Input: part model. Units: mm. Frame: model coordinates. A direction names the side the tool comes from. Round coordinates to 2 decimals unless told otherwise and drop trailing zeros. Write each loop counter-clockwise with the first axis right and the second up, starting at its lowest first coordinate (ties: lowest second). Pieces come first, ordered by that corner, then holes. Notation, with made-up numbers: (68, 26.5) -> (77, 26.5) arc R33 ccw to (77, 58.5) -> close; hole circle Ø10 at (68, 43.5). An arc over 180 degrees is marked (long way). Write item = value, one per line. Start each with the question number.
```python
from build123d import *

# Parameters (mm, degrees)
SHAFTSKETCH_R           = 6.5
BEARINGHOLEPAD_DEPTH    = 5
SHAFT1SKETCH_R          = 7.5
OBJ1 = 5
PIN1SKETCH_R            = 2
PIN1PAD_DEPTH           = 10
PIN2SKETCH_R            = 2
PIN2PAD_DEPTH           = 10
OBJ2    = 15


with BuildPart() as part:
    # ShaftSketch → bearingholePad (new body)
    with BuildSketch(Plane.XY):
        Circle(SHAFTSKETCH_R)
    extrude(amount=BEARINGHOLEPAD_DEPTH)

    with BuildSketch(Plane.XY.offset(5)):
        Circle(SHAFT1SKETCH_R)
    extrude(amount=OBJ1)

    # Pin1Sketch → Pin1Pad (join)
    with BuildSketch(Plane.XY.offset(5)):
        with Locations((1.75, 0)):
            Circle(PIN1SKETCH_R)
    extrude(amount=PIN1PAD_DEPTH)

    # Pin2Sketch → Pin2Pad (join)
    with BuildSketch(Plane.XY.offset(5)):
        with Locations((3.5, 0)):
            Circle(PIN2SKETCH_R)
    extrude(amount=PIN2PAD_DEPTH)

    with BuildSketch(Plane.XY):
        with BuildLine():
            ThreePointArc((-0.979796, 2.3), (0, -2.5), (0.979796, 2.3))
            Line((-0.979796, 2.3), (0.979796, 2.3))
        make_face()
    extrude(amount=OBJ2, mode=Mode.SUBTRACT)


solid = part.part
```
1. Section A-A (y = 0). Output: boundary loops of the cut face in (x, z).
2. Pin query (flat end, axial travel): P1, Ø6.5, axis at x = 0, y = 0, coming from the +Z side; P2, Ø3, axis at x = 5.5, z = 12, coming from the -Y side; P3, Ø1.6, axis at x = 0, z = 4, coming from the -Y side; P4, Ø5, axis at x = -0.5, z = 13, coming from the +Y side. Return the tip coordinate at first contact, or that it passes through.
3. Line query: line 1 along Y through (x, z) = (0, 9.75); line 2 along Y through (x, z) = (0, 4.5); line 3 along Z through (x, y) = (-4.75, 3). Output: solid intervals per line, ascending.
4. Section D-D (x = -6). Output: boundary loops of the cut face in (y, z), then the cut area to 3 significant figures.
5. Reachability of faces 4 (the cylindrical face through (2.077, -1.973, 12.465)), 5 (the cylindrical face through (-5.158, -3.955, 2.465)), 6 (the cylindrical face through (2.09, 1.97, 12.46)), 7 (the flat face through (0, 2.3, 5)) from +Z, -Z, +X, -X, +Y, -Y: full face, straight path, thin tool, end or side. Return the list, or none.
6. Section C-C (z = 7.5). Output: boundary loops of the cut face in (x, y).
7. Section B-B (x = 0). Output: boundary loops of the cut face in (y, z).
8. Mould query, pull axis Y, two halves, no side actions, for faces 1 (the cylindrical face through (5.5, -0.06, 12.46)), 2 (the cylindrical face through (2.31, -0.955, 5.728)), 3 (the flat face through (3, 0, 0)). Classes: pulls with the +Y half, pulls with the -Y half, needs draft (parallel to the pull), parting line crosses it, or undercut.
Check sheet entries:
q1.outline = (-7.5, 5) -> (-6.5, 5) -> (-6.5, 0) -> (-2.5, 0) -> (-2.5, 10) -> (-7.5, 10) -> close; (2.5, 0) -> (6.5, 0) -> (6.5, 5) -> (7.5, 5) -> (7.5, 10) -> (5.5, 10) -> (5.5, 15) -> (2.5, 15) -> close
q2.P1 = 15
q2.P2 = -1.94
q2.P3 = -6.5
q2.P4 = 2
q3.line_1 = -7.5 to -2.5, 2.3 to 7.5
q3.line_2 = -6.5 to -2.5, 2.3 to 6.5
q3.line_3 = 0 to 10
q4.outline = (-4.5, 5) -> (-2.5, 5) -> (-2.5, 0) -> (2.5, 0) -> (2.5, 5) -> (4.5, 5) -> (4.5, 10) -> (-4.5, 10) -> close
q4.area = 70.0 mm2
q5.face_4 = +Z, -Y
q5.face_5 = -Z
q5.face_6 = +Z, +Y
q5.face_7 = +Z, -Z
q6.outline = circle Ø15 at (0, 0); hole (-0.98, 2.3) arc R2.5 ccw (long way) to (0.98, 2.3) -> close
q7.outline = (-7.5, 5) -> (-6.5, 5) -> (-6.5, 0) -> (-2.5, 0) -> (-2.5, 10) -> (-7.5, 10) -> close; (2.3, 0) -> (6.5, 0) -> (6.5, 5) -> (7.5, 5) -> (7.5, 10) -> (2.3, 10) -> close
q8.face_1 = parting line crosses it
q8.face_2 = undercut
q8.face_3 = needs draft
